from build123d import *

# Parameters (mm, degrees)
F0_R     = 17.421619
F1_DEPTH = 7.62
F3_DEPTH = 7.62
F4_SIZE  = 0.762
F5_R     = 6.35
F6_DEPTH = 25.4


with BuildPart() as f1:
    # F0 (on Front) → F1 (new body)
    with BuildSketch(Plane.XZ):
        Circle(F0_R)
    extrude(amount=F1_DEPTH)

    # F2 (on face) → F3 (join, through all)
    with BuildSketch(Plane(origin=(0, 0, 0), x_dir=(-1, 0, 0), z_dir=(0, 1, 0))):
        Polygon((-17.235463, -2.54), (-17.235463, 2.54), (-21.634872, 0), align=None)
        Polygon((-20.575986, -6.685543), (-15.606996, -7.741735), (-17.176803, -2.910368), align=None)
        Polygon((-17.502979, -12.716659), (-12.450808, -12.185654), (-15.436757, -8.075848), align=None)
        Polygon((-12.716659, -17.502979), (-8.075848, -15.436757), (-12.185654, -12.450808), align=None)
        Polygon((-6.685543, -20.575986), (-2.910368, -17.176803), (-7.741735, -15.606996), align=None)
        Polygon((0, -21.634872), (2.54, -17.235463), (-2.54, -17.235463), align=None)
        Polygon((6.685543, -20.575986), (7.741735, -15.606996), (2.910368, -17.176803), align=None)
        Polygon((12.716659, -17.502979), (12.185654, -12.450808), (8.075848, -15.436757), align=None)
        Polygon((17.502979, -12.716659), (15.436757, -8.075848), (12.450808, -12.185654), align=None)
        Polygon((20.575986, -6.685543), (17.176803, -2.910368), (15.606996, -7.741735), align=None)
        Polygon((21.634872, 0), (17.235463, 2.54), (17.235463, -2.54), align=None)
        Polygon((20.575986, 6.685543), (15.606996, 7.741735), (17.176803, 2.910368), align=None)
        Polygon((17.502979, 12.716659), (12.450808, 12.185654), (15.436757, 8.075848), align=None)
        Polygon((12.716659, 17.502979), (8.075848, 15.436757), (12.185654, 12.450808), align=None)
        Polygon((6.685543, 20.575986), (2.910368, 17.176803), (7.741735, 15.606996), align=None)
        Polygon((0, 21.634872), (-2.54, 17.235463), (2.54, 17.235463), align=None)
        Polygon((-6.685543, 20.575986), (-7.741735, 15.606996), (-2.910368, 17.176803), align=None)
        Polygon((-12.716659, 17.502979), (-12.185654, 12.450808), (-8.075848, 15.436757), align=None)
        Polygon((-17.502979, 12.716659), (-15.436757, 8.075848), (-12.450808, 12.185654), align=None)
        Polygon((-20.575986, 6.685543), (-17.176803, 2.910368), (-15.606996, 7.741735), align=None)
    extrude(amount=-F3_DEPTH)

    # F4
    f4_edges = [f1.edges().sort_by_distance(p)[0] for p in [
        (-6.685543, -3.81, 20.575986),
        (0, -3.81, 21.634872),
        (6.685543, -3.81, 20.575986),
        (12.716659, -3.81, 17.502979),
        (17.502979, -3.81, 12.716659),
        (20.575986, -3.81, 6.685543),
        (21.634872, -3.81, 0),
        (20.575986, -3.81, -6.685543),
        (-12.716659, -3.81, 17.502979),
        (-17.502979, -3.81, 12.716659),
        (-20.575986, -3.81, 6.685543),
        (-21.634872, -3.81, 0),
        (-20.575986, -3.81, -6.685543),
        (-17.502979, -3.81, -12.716659),
        (-12.716659, -3.81, -17.502979),
        (17.502979, -3.81, -12.716659),
        (-6.685543, -3.81, -20.575986),
        (0, -3.81, -21.634872),
        (6.685543, -3.81, -20.575986),
        (12.716659, -3.81, -17.502979),
    ]]
    chamfer(f4_edges, length=F4_SIZE)

    # F5 (on face) → F6 (cut)
    with BuildSketch(Plane.XZ.offset(7.62)):
        Circle(F5_R)
    extrude(amount=-F6_DEPTH, mode=Mode.SUBTRACT)


solid = f1.part
Verification items for the finished model (mm, model axes). A direction names the side the tool comes from. Give positions to 0.01 mm unless a question says otherwise; leave off trailing zeros. Loops run counter-clockwise (first coordinate to the right, second up) from the corner with the lowest first, then second, coordinate; pieces in that order, holes last. Notation, with made-up numbers: (73.25, 39) - (113.25, 39) arc R27 ccw to (113.25, 73) - close; hole circle Ø3 at (79, -30). An arc over 180 degrees is marked (long way). Write item = value, one per line. Start each with the question number.
Q1. Cross-section at B-B, the plane x = -10. Enter the section's corners in (y, z).
Q2. Cross-section at C-C, the plane x = 9. Enter the section's corners in (y, z), and give its area (3 significant figures).
Q3. Depth check by flat-ended pin: P1, Ø6, axis at x = -7, z = -1, coming from the +Y side; P2, Ø3, axis at x = -11, y = -2, coming from the -Z side; P3, Ø1.5, axis at x = 4.5, y = -2, coming from the +Z side; P4, Ø4, axis at y = -1, z = 10.5, coming from the +X side. Enter the tip coordinate at first touch or a pass-through.
Q4. Mould release check, pull along Z, two halves, no side actions. Record for faces 4 (the face through (-1.445, -3.757, -19.131)), 5 (the face through (10.021, -3.757, 16.303)), 6 (the face through (-16.303, -3.757, 10.021)): released by +Z, released by -Z, zero draft, split by the parting line, or undercut.
Q5. Cross-section at A-A, the plane x = -1.5. Enter the section's corners in (y, z).
Q6. Thickness scan on line 1 (Z direction, x = 0, y = -5.5); line 2 (Z direction, x = -19, y = -0.75); line 3 (X direction, y = -7, z = 3). Record the ranges inside material, lowest first.
Q7. Tool access check on faces 1 (the face through (-1.476, -3.757, 19.079)), 2 (the face through (18.6, -3.76, -4.49)), 3 (the face through (4.537, -3.757, -18.642)). Record the directions out of +Z, -Z, +X, -X, +Y, -Y that give a thin tool (end or side, any length) a straight path to the whole face; none if there is none.
Answer key:
q1.outline = (-7.62, -16.29) - (0, -16.29) - (0, 16.29) - (-7.62, 16.29) - close
q2.outline = (-7.62, -15.85) - (0, -15.85) - (0, 15.85) - (-7.62, 15.85) - close
q2.area = 242 mm^2
q3.P1 = 0
q3.P2 = -17.19
q3.P3 = 19.28
q3.P4 = 17.19
q4.face_4 = released by -Z
q4.face_5 = released by +Z
q4.face_6 = undercut
q5.outline = (-7.62, -19.04) - (0, -19.04) - (0, -6.17) - (-7.62, -6.17) - close; (-7.62, 6.17) - (0, 6.17) - (0, 19.04) - (-7.62, 19.04) - close
q6.line_1 = -20.97 to -6.35, 6.35 to 20.97
q6.line_2 = -7.02 to -4.94, -1.52 to 1.52, 4.94 to 7.02
q6.line_3 = -17.26 to -5.6, 5.6 to 17.26
q7.face_1 = +Z, +Y, -Y
q7.face_2 = +X, +Y, -Y
q7.face_3 = -Z, +Y, -Y
